from build123d import *

# Parameters (mm, degrees)
SKETCH1_W               = 34.925
SKETCH1_H               = 34.925
SKETCH1_W_2             = 30.9626
SKETCH1_H_2             = 30.9626
BOSS_EXTRUDE1_DEPTH     = 219.075
SKETCH2_W               = 76.400000108
SKETCH2_H               = 6.550000108
CUT_EXTRUDE1_DEPTH      = 223.527639084
CUT_EXTRUDE3_DEPTH      = 221.462544296
CUT_EXTRUDE3_DEPTH_BACK = 221.462544296
SKETCH5_R               = 1.56250005
SKETCH6_R               = 1.56250005
CUT_EXTRUDE5_DEPTH      = 223.527639084


with BuildPart() as part:
    # Sketch1 → Boss-Extrude1 (new, symmetric)
    with BuildSketch(Plane(origin=(0, 0, 0), x_dir=(0, 0, -1), z_dir=(1, 0, 0))):
        Rectangle(SKETCH1_W, SKETCH1_H)
        Rectangle(SKETCH1_W_2, SKETCH1_H_2, mode=Mode.SUBTRACT)
    extrude(amount=BOSS_EXTRUDE1_DEPTH, both=True)

    # Sketch2 → Cut-Extrude1 (cut, through all)
    with BuildSketch(Plane(origin=(0, 17.4625, 0), x_dir=(1, 0, 0), z_dir=(0, 1, 0))):
        Rectangle(SKETCH2_W, SKETCH2_H)
    extrude(amount=-CUT_EXTRUDE1_DEPTH, mode=Mode.SUBTRACT)

    # Sketch5 → Cut-Extrude3 (cut, two sides: drawn at the far end of the back side and taken through both)
    with BuildSketch(Plane.XY.offset(-CUT_EXTRUDE3_DEPTH_BACK)):
        with Locations((-203.175, 9.5)):
            Circle(SKETCH5_R)
        with Locations((-193.675, 0)):
            Circle(SKETCH5_R)
        with Locations((-203.175, -9.5)):
            Circle(SKETCH5_R)
        with Locations((-212.675, 0)):
            Circle(SKETCH5_R)
        with Locations((212.675, 0)):
            Circle(SKETCH5_R)
        with Locations((203.175, -9.5)):
            Circle(SKETCH5_R)
        with Locations((193.675, 0)):
            Circle(SKETCH5_R)
        with Locations((203.175, 9.5)):
            Circle(SKETCH5_R)
    extrude(amount=CUT_EXTRUDE3_DEPTH + CUT_EXTRUDE3_DEPTH_BACK, mode=Mode.SUBTRACT)

    # Sketch6 → Cut-Extrude5 (cut, through all)
    with BuildSketch(Plane.XY.offset(17.4625)):
        with Locations((-101.6, 9.5)):
            Circle(SKETCH6_R)
        with Locations((-92.1, 0)):
            Circle(SKETCH6_R)
        with Locations((-101.6, -9.5)):
            Circle(SKETCH6_R)
        with Locations((-111.1, 0)):
            Circle(SKETCH6_R)
    cut_extrude5 = extrude(amount=-CUT_EXTRUDE5_DEPTH, mode=Mode.SUBTRACT)

    # Mirror1: Cut-Extrude5 across plane
    add(cut_extrude5.mirror(Plane(origin=(0, 0, 0), x_dir=(0, 0, 1), z_dir=(1, 0, 0))), mode=Mode.SUBTRACT)


solid = part.part
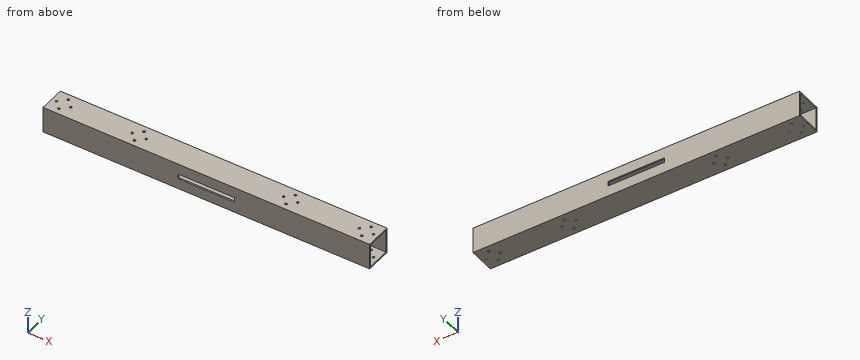
Read the model definition and answer for the solid it produces. Units are mm, in the model's axes. Give positions to 0.01 mm unless a question says otherwise; leave off trailing zeros. Write each loop counter-clockwise with the first axis right and the second up, starting at its lowest first coordinate (ties: lowest second). Pieces come first, ordered by that corner, then holes. Notation, with made-up numbers: (68, -9) - (81, -9) arc R24 cw to (81, 20) - close; hole circle Ø7 at (-8, -5). An arc over 180 degrees is marked (long way). Return JSON: item names as keys, results as strings.
Q1. A cutting plane is placed at B-B, the plane z = -11. Determine the outline of the cut face in (x, y) (1 decimal), and give its area (3 significant figures).
Reply:
{"outline": "(-219.1, -17.5) - (219.1, -17.5) - (219.1, -15.5) - (-219.1, -15.5) - close; (-219.1, 15.5) - (219.1, 15.5) - (219.1, 17.5) - (-219.1, 17.5) - close", "area": "1,740 mm²"}
Q2. A cutting plane is placed at A-A, the plane x = -28. Determine the outline of the cut face in (y, z) (1 decimal).
Reply:
{"outline": "(-17.5, -17.5) - (17.5, -17.5) - (17.5, -3.3) - (15.5, -3.3) - (15.5, -15.5) - (-15.5, -15.5) - (-15.5, -3.3) - (-17.5, -3.3) - close; (-17.5, 3.3) - (-15.5, 3.3) - (-15.5, 15.5) - (15.5, 15.5) - (15.5, 3.3) - (17.5, 3.3) - (17.5, 17.5) - (-17.5, 17.5) - close"}
Q3. Given P1, Ø2.5, axis at x = 212.675, y = 0, coming from the +Z side, flat-ended and moving along its own axis, determine where the tip first touches the part or whether it passes through.
Reply:
{"P1": "through"}
Q4. A cutting plane is placed at C-C, the plane x = -117. Determine the outline of the cut face in (y, z).
Reply:
{"outline": "(-17.46, -17.46) - (17.46, -17.46) - (17.46, 17.46) - (-17.46, 17.46) - close; hole (-15.48, -15.48) - (15.48, -15.48) - (15.48, 15.48) - (-15.48, 15.48) - close"}
Q5. Consider line 1 along Z through (x, y) = (-100, 12.5); line 2 along Y through (x, z) = (-101, 16). Determine where each line is inside the solid, lowest interval first. Write a range as [from, to].
Reply:
{"line 1": "[-17.46, -15.48], [15.48, 17.46]", "line 2": "[-17.46, -10.94], [-8.06, 8.06], [10.94, 17.46]"}
